Geometry: see drawing. Coordinates: mm, zero at the bounding-box minimum. Coordinates: 2 decimals unless noted, no trailing zeros. Write each loop counter-clockwise with the first axis right and the second up, starting at its lowest first coordinate (ties: lowest second). Pieces come first, ordered by that corner, then holes.
1) Section query D-D (z = 69.5). Output: boundary loops of the cut face in (x, y).
2) Section query A-A (y = 50). Output: boundary loops of the cut face in (x, z), then the cut area to 3 significant figures.
3) Section query C-C (z = 14.5). Output: boundary loops of the cut face in (x, y), then the cut area to 3 significant figures.
4) Line query: L1, parallel to Y at x = 50, z = 91; L2, parallel to Y at x = 47, z = 31.5; L3, parallel to X at y = 73, z = 26.5 (1 decimal). Output: solid intervals per line, ascending.
5) Draft query along X for the marked faces 1, 2, 3 and 4. Return one class per face: pulls with the +X half, pulls with the -X half, needs draft (parallel to the pull), parting line crosses it, or undercut.
6) Pin query (flat end, axial travel): pin 1 Ø4 at (y, z) = (52.5, 41.5) entering from -X; pin 2 Ø8 at (x, y) = (57.5, 53.5) entering from +Z. Return the tip coordinate at first contact, or that it passes through.
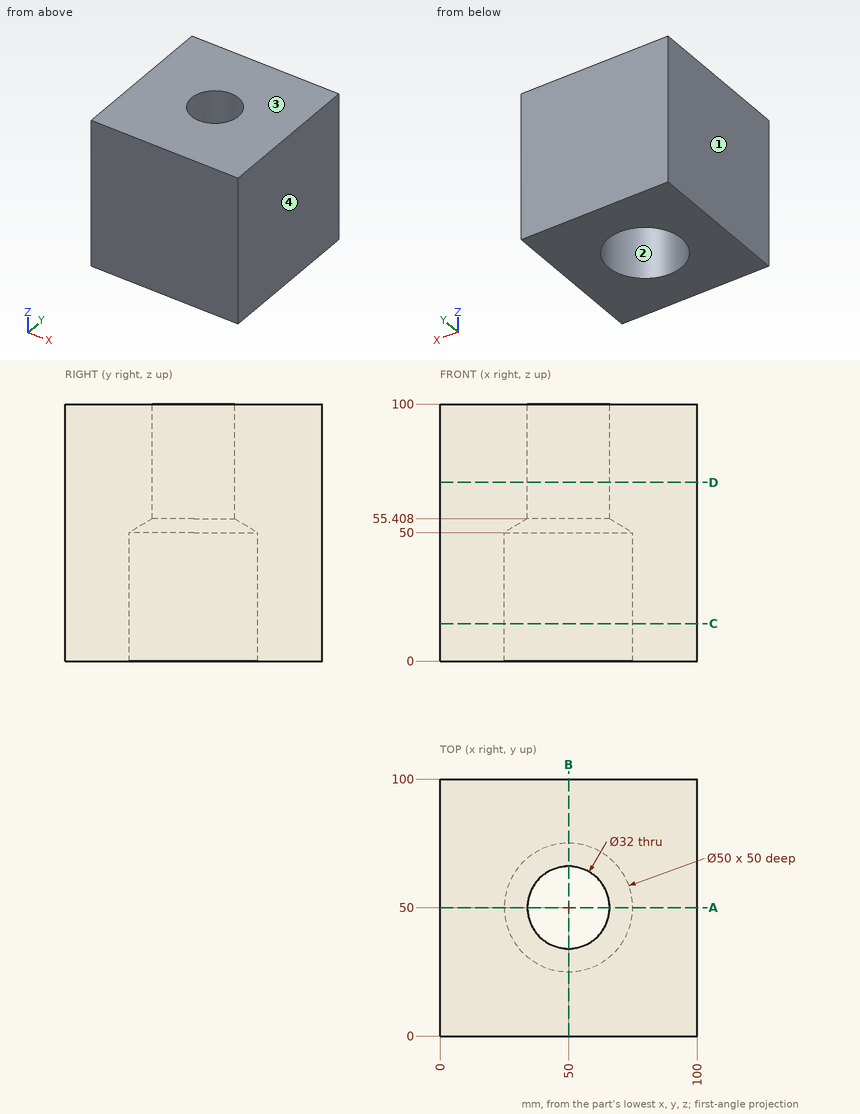
Answer:
1. outline: (0, 0) - (100, 0) - (100, 100) - (0, 100) - close; hole circle Ø32 at (50, 50)
2. outline: (0, 0) - (25, 0) - (25, 50) - (34, 55.41) - (34, 100) - (0, 100) - close; (66, 55.41) - (75, 50) - (75, 0) - (100, 0) - (100, 100) - (66, 100) - close
2. area: 5,850 mm2
3. outline: (0, 0) - (100, 0) - (100, 100) - (0, 100) - close; hole circle Ø50 at (50, 50)
3. area: 8,040 mm2
4. L1: y = 0 to 34, 66 to 100
4. L2: y = 0 to 25.18, 74.82 to 100
4. L3: x = 0 to 40.2, 59.8 to 100
5. face 1: pulls with the -X half
5. face 2: undercut
5. face 3: needs draft
5. face 4: pulls with the +X half
6. pin 1: stops at x = 0
6. pin 2: passes through
